from build123d import *

# Parameters (mm, degrees)
SKETCH_1_R          = 4.25
EXTRUDE_1_DEPTH     = 5
SKETCH_2_R          = 2.5
EXTRUDE_2_DEPTH     = 20
CUT_EXTRUDE_1_DEPTH = 2


with BuildPart() as part:
    # ｽｹｯﾁ1 → ﾎﾞｽ - 押し出し1 (new body)
    with BuildSketch(Plane.XY):
        Circle(SKETCH_1_R)
    extrude(amount=EXTRUDE_1_DEPTH)

    # ｽｹｯﾁ2 → ﾎﾞｽ - 押し出し2 (add)
    with BuildSketch(Plane.XY.offset(5)):
        Circle(SKETCH_2_R)
    extrude(amount=EXTRUDE_2_DEPTH)

    # ｽｹｯﾁ3 → ｶｯﾄ - 押し出し1 (cut)
    with BuildSketch(Plane(origin=(0, 0, 0), x_dir=(-1, 0, 0), z_dir=(0, 0, -1))):
        Polygon((2.481247226, -1.110941893), (2.202727514, 1.593352185), (-0.278519712, 2.704294077), (-2.481247226, 1.110941893), (-2.202727514, -1.593352185), (0.278519712, -2.704294077), align=None)
    extrude(amount=-CUT_EXTRUDE_1_DEPTH, mode=Mode.SUBTRACT)


solid = part.part
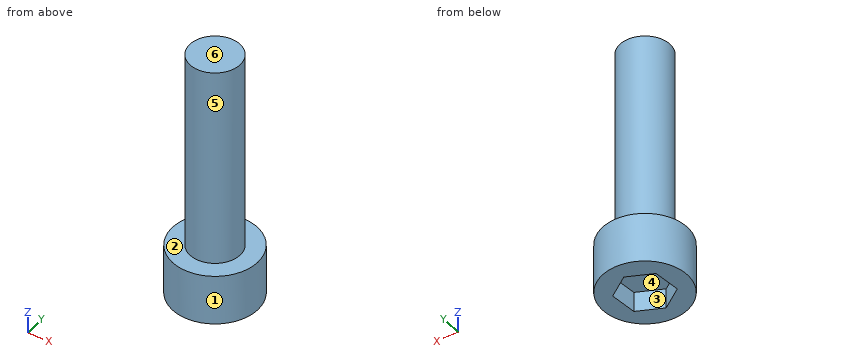
Verification items for the finished model (mm, model axes). Face numbers are marked on the shaded views. A direction names the side the tool comes from. Coordinates: 2 decimals unless noted, no trailing zeros. Order: outer loops, then holes, each group sorted by start corner. A loop starts at its lowest first (then second) coordinate and runs counter-clockwise, first axis right, second up. Notation, with made-up numbers: M -6.75,57 L 10.25,57 A8 cw 10.25,63 Z; hole C 89.25,-17 d1. An arc over 180 degrees is marked long. Return JSON: item names as keys, results as strings.
1) Cross-section at A-A, the plane x = 1.5. Record the boundary of the cut face in (y, z), and give its area (3 significant figures).
Answer list:
{"outline": "M -3.98,0 L -1.91,0 L -1.91,2 L 1.82,2 L 1.82,0 L 3.98,0 L 3.98,5 L 2,5 L 2,25 L -2,25 L -2,5 L -3.98,5 Z", "area": "112 mm2"}
2) Release check for a two-part mould opening along X. For the marked faces 4, 5 and 6 record: +X half, -X half, draft (parallel to the pull), parting line (faces both ways), or undercut.
Answer list:
{"face 4": "undercut", "face 5": "parting line", "face 6": "draft"}
3) Cross-section at B-B, the plane y = 2.25. Record the boundary of the cut face in (x, z), and give its area (3 significant figures).
Answer list:
{"outline": "M -3.61,0 L -0.74,0 L -0.74,2 L 0.91,2 L 0.91,0 L 3.61,0 L 3.61,5 L 1.09,5 L 1.09,25 L -1.09,25 L -1.09,5 L -3.61,5 Z", "area": "76.4 mm2"}
4) Gauge pin test, flat ends, axial feed: pin 1 (1.5 mm diameter, centred on x = -2.5, z = 20, fed in from +Y); pin 2 (5 mm diameter, centred on y = 2, z = 19, fed in from -X); pin 3 (2 mm diameter, centred on x = -2, z = 17.5, fed in from +Y). Record the tip position at first contact, or that the pin passes through.
Answer list:
{"pin 1": "y = 1.79", "pin 2": "x = -2.5", "pin 3": "y = 2.29"}
5) Thickness scan on L1, parallel to Z at x = 2.25, y = -2; L2, parallel to Z at x = -1.5, y = -1; L3, parallel to Y at x = 1.25, z = 1.5. Record the ranges inside material, lowest first. Write a range as [from, to].
Answer list:
{"L1": "[0, 5]", "L2": "[2, 25]", "L3": "[-4.06, -2.02], [2, 4.06]"}
6) Cross-section at C-C, the plane z = 11.5. Record the boundary of the cut face in (x, y).
Answer list:
{"outline": "C 0,0 d5"}
7) Access from +Z, -Z, +X, -X, +Y, -Y to the whole of each face (thin tool, end or side, straight path). Record for the marked faces 1, 2 and 3.
Answer list:
{"face 1": "+Z, -Z", "face 2": "+Z", "face 3": "-Z"}
8) Cross-section at D-D, the plane x = -3.25. Record the boundary of the cut face in (y, z), and give its area (3 significant figures).
Answer list:
{"outline": "M -2.74,0 L 2.74,0 L 2.74,5 L -2.74,5 Z", "area": "27.4 mm2"}
